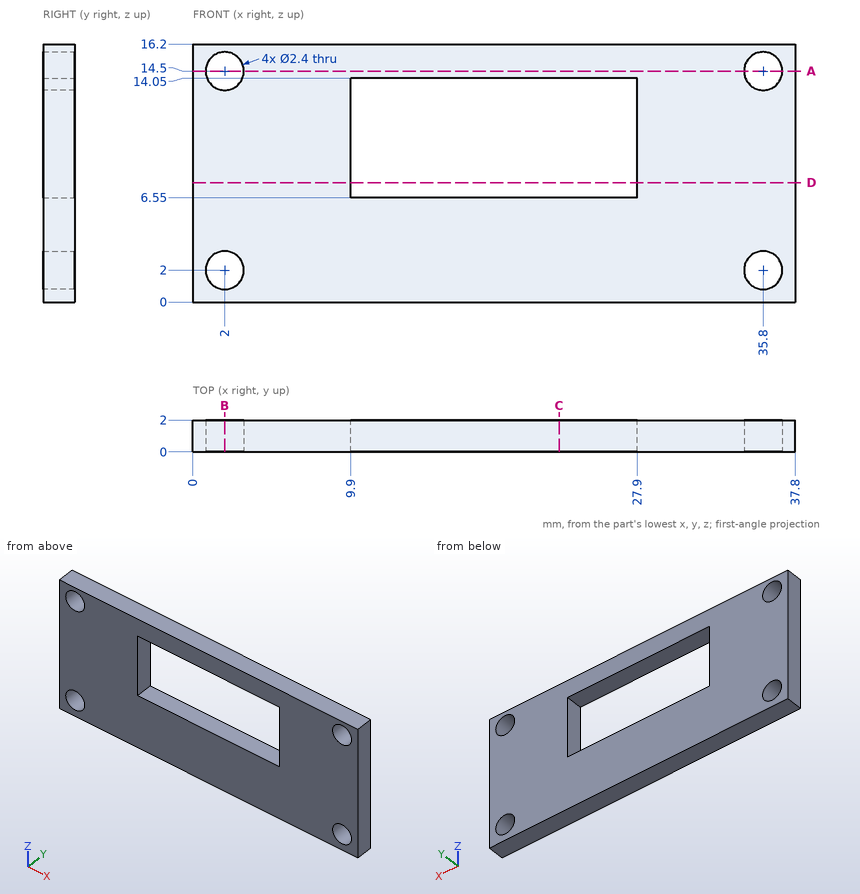
Drawing for the job (mm, zero at the part's lowest x, y, z). Round coordinates to 2 decimals unless told otherwise and drop trailing zeros. Write each loop counter-clockwise with the first axis right and the second up, starting at its lowest first coordinate (ties: lowest second). Pieces come first, ordered by that corner, then holes. Notation, with made-up numbers: M 5,28.25 L 62,28.25 A19 cw 62,41.25 Z; hole C 7.25,-21.75 d5. An arc over 180 degrees is marked long. Answer as a JSON object with one key per item and string values. Group by question number.
(1) Cut at A-A (z = 14.5). Give the cut face in (x, y).
(2) Cut at B-B (x = 2). Give the cut face in (y, z).
(3) Drill centre lines: L1, parallel to X at y = 0.6, z = 14.5; L2, parallel to Z at x = 2, y = 0.55; L3, parallel to Z at x = 15.5, y = 0.3. Where is each one in solid material? Low to high.
(4) Cut at D-D (z = 7.5). Give the cut face in (x, y).
(5) Flat gauge pins, fed straight in: pin 1 (1.5 mm diameter, centred on x = 4.5, z = 3.5, fed in from -Y); pin 2 (1.4 mm diameter, centred on x = 2, z = 2, fed in from +Y). Where does each tip first touch, or does it go through?
(6) Cut at C-C (x = 23). Give the cut face in (y, z).
Responses:
{
 "1": {"outline": "M 0,0 L 0.8,0 L 0.8,2 L 0,2 Z; M 3.2,0 L 34.6,0 L 34.6,2 L 3.2,2 Z; M 37,0 L 37.8,0 L 37.8,2 L 37,2 Z"},
 "2": {"outline": "M 0,0 L 2,0 L 2,0.8 L 0,0.8 Z; M 0,3.2 L 2,3.2 L 2,13.3 L 0,13.3 Z; M 0,15.7 L 2,15.7 L 2,16.2 L 0,16.2 Z"},
 "3": {"L1": "x = 0 to 0.8, 3.2 to 34.6, 37 to 37.8", "L2": "z = 0 to 0.8, 3.2 to 13.3, 15.7 to 16.2", "L3": "z = 0 to 6.55, 14.05 to 16.2"},
 "4": {"outline": "M 0,0 L 9.9,0 L 9.9,2 L 0,2 Z; M 27.9,0 L 37.8,0 L 37.8,2 L 27.9,2 Z"},
 "5": {"pin 1": "stops at y = 0", "pin 2": "passes through"},
 "6": {"outline": "M 0,0 L 2,0 L 2,6.55 L 0,6.55 Z; M 0,14.05 L 2,14.05 L 2,16.2 L 0,16.2 Z"}
}
